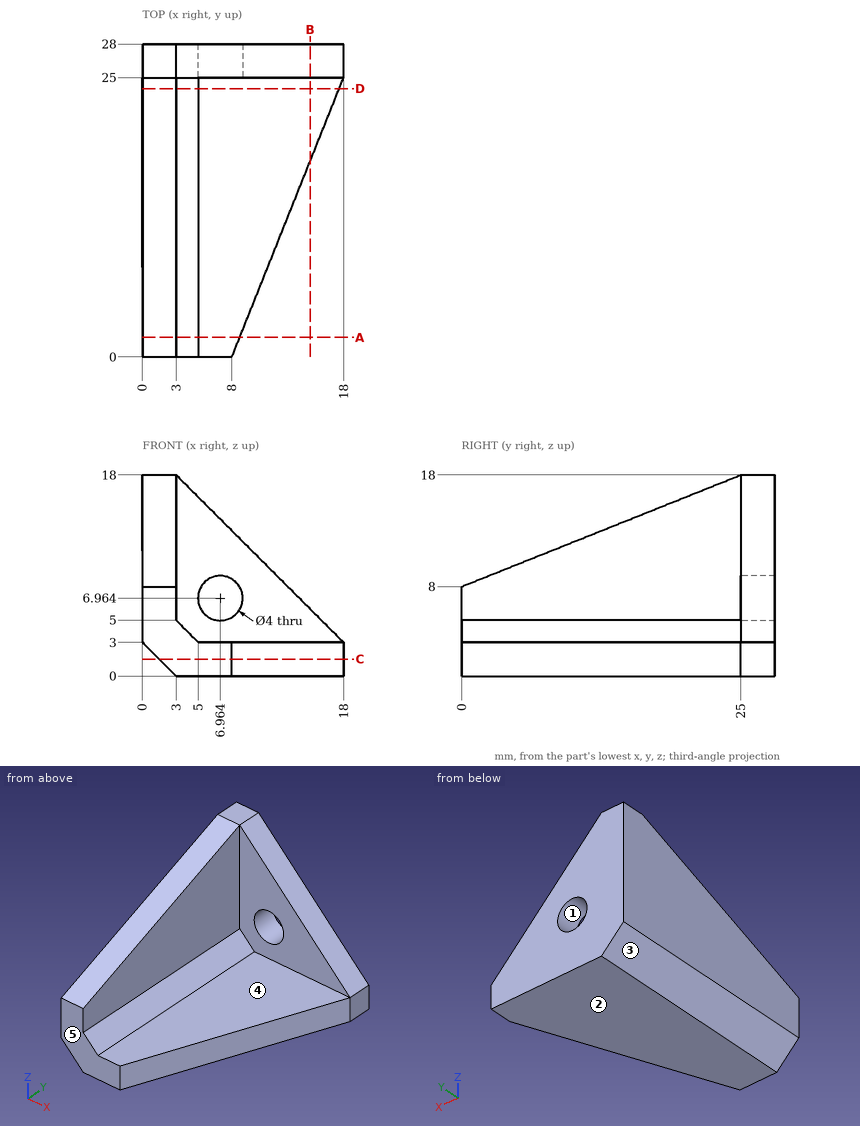
Here's the drawing with two shaded views (mm, measured from the low corner). I have some questions. A direction names the side the tool comes from. Coordinates: 2 decimals unless noted, no trailing zeros. Loops run counter-clockwise (first coordinate to the right, second up) from the corner with the lowest first, then second, coordinate; pieces in that order, holes last. Notation, with made-up numbers: M 10,54.25 L 53,54.25 A32 cw 53,87.25 Z; hole C 85,0 d1. An arc over 180 degrees is marked long. Return JSON: item names as keys, results as strings. Group by question number.
Item 1: Imagine slicing it at C-C (z = 1.5). Please give me the cut outline in (x, y), and give its area (3 significant figures).
Item 2: If I drill on L1, parallel to X at y = 14.75, z = 11.5; L2, parallel to Z at x = 8.5, y = 25.5 (1 decimal), over which ranges is the centre line in solid material (lowest first)? Write a range as from..to.
Item 3: On a 3-axis mill with a long thin cutter (end or side, diameter ignored), from which of +Z, -Z, +X, -X, +Y, -Y can I reach the whole of each face in a straight line? I mean the marked faces 4 and 5. Say none if no direction works.
Item 4: Imagine slicing it at B-B (x = 15). Please give me the cut outline in (y, z), and give its area (3 significant figures).
Item 5: Thinking about a two-plate mould opening in X: for the marked faces 1, 2 and 3, which applies, released by +X, released by -X, zero draft, split by the parting line, or undercut?
Item 6: I'm going to push flat-ended pins straight in: pin 1 Ø1.5 at (x, y) = (3.5, 21.5) entering from +Z; pin 2 Ø3 at (y, z) = (17.5, 4) entering from +X; pin 3 Ø4 at (y, z) = (18.5, 13.5) entering from +X. Where does each tip first touch, or does it pass through?
Item 7: Imagine slicing it at A-A (y = 1.75). Please give me the cut outline in (x, z).
Item 8: Imagine slicing it at D-D (y = 24). Please give me the cut outline in (x, z).
Verdict:
{
 "1": {"outline": "M 1.5,0 L 8,0 L 18,25 L 18,28 L 1.5,28 Z", "area": "337 mm^2"},
 "2": {"L1": "x = 0..3", "L2": "z = 0..5.7, 8.2..12.5"},
 "3": {"face 4": "+Z, +X, -Y", "face 5": "+Z, -Z, +X, -X, -Y"},
 "4": {"outline": "M 17.5,0 L 28,0 L 28,6 L 25,6 L 25,3 L 17.5,3 Z", "area": "40.5 mm^2"},
 "5": {"face 1": "undercut", "face 2": "zero draft", "face 3": "released by -X"},
 "6": {"pin 1": "stops at z = 16.82", "pin 2": "stops at x = 15.45", "pin 3": "stops at x = 3"},
 "7": {"outline": "M 0,3 L 3,0 L 8.7,0 L 8.7,3 L 5,3 L 3,5 L 3,8.7 L 0,8.7 Z"},
 "8": {"outline": "M 0,3 L 3,0 L 17.6,0 L 17.6,3 L 5,3 L 3,5 L 3,17.6 L 0,17.6 Z"}
}
